from build123d import *

# Parameters (mm, degrees)
SKETCH1_W           = 50
SKETCH1_H           = 51
BOSS_EXTRUDE1_DEPTH = 3
SKETCH2_W           = 50
SKETCH2_H           = 3
BOSS_EXTRUDE2_DEPTH = 50
FILLET1_R           = 2
CHAMFER1_SIZE       = 5
CUT_EXTRUDE1_DEPTH  = 50
SKETCH4_R           = 12.55
SKETCH4_R_2         = 2.1
CUT_EXTRUDE2_DEPTH  = 50
BOSS_EXTRUDE3_DEPTH = 3


with BuildPart() as part:
    # Sketch1 → Boss-Extrude1 (new body)
    with BuildSketch(Plane.XY):
        Rectangle(SKETCH1_W, SKETCH1_H)
    extrude(amount=BOSS_EXTRUDE1_DEPTH)

    # Sketch2 → Boss-Extrude2 (add)
    with BuildSketch(Plane.XY.offset(3)):
        with Locations((0, -24)):
            Rectangle(SKETCH2_W, SKETCH2_H)
    extrude(amount=BOSS_EXTRUDE2_DEPTH)

    # Fillet1
    fillet1_edges = [part.edges().sort_by_distance(p)[0] for p in [
        (0, -22.5, 3),
        (0, -25.5, 0),
    ]]
    fillet(fillet1_edges, radius=FILLET1_R)

    # Chamfer1
    chamfer1_edges = [part.edges().sort_by_distance(p)[0] for p in [
        (-25, -24, 53),
        (25, -24, 53),
        (-25, 25.5, 1.5),
        (25, 25.5, 1.5),
    ]]
    chamfer(chamfer1_edges, length=CHAMFER1_SIZE)

    # Sketch3 → Cut-Extrude1 (cut)
    with BuildSketch(Plane(origin=(0, -22.5, 0), x_dir=(1, 0, 0), z_dir=(0, 1, 0))):
        with BuildLine():
            Line((-17.1, -42), (-17.1, -12))
            ThreePointArc((-17.1, -12), (-15, -9.9), (-12.9, -12))
            Line((-12.9, -12), (-12.9, -42))
            ThreePointArc((-12.9, -42), (-15, -44.1), (-17.1, -42))
        make_face()
        with BuildLine():
            Line((12.9, -42), (12.9, -12))
            ThreePointArc((12.9, -12), (15, -9.9), (17.1, -12))
            Line((17.1, -12), (17.1, -42))
            ThreePointArc((17.1, -42), (15, -44.1), (12.9, -42))
        make_face()
    extrude(amount=-CUT_EXTRUDE1_DEPTH, mode=Mode.SUBTRACT)

    # Sketch4 → Cut-Extrude2 (cut)
    with BuildSketch(Plane.XY.offset(3)):
        with Locations((0, 4.5)):
            Circle(SKETCH4_R)
        with Locations((0, 22)):
            Circle(SKETCH4_R_2)
        with Locations((0, -13)):
            Circle(SKETCH4_R_2)
        with Locations((17.5, 4.5)):
            Circle(SKETCH4_R_2)
        with Locations((-17.5, 4.5)):
            Circle(SKETCH4_R_2)
    extrude(amount=-CUT_EXTRUDE2_DEPTH, mode=Mode.SUBTRACT)

    # Sketch5 → Boss-Extrude3 (add)
    with BuildSketch(Plane.ZY.offset(25)):
        with BuildLine():
            Line((3, -2.5), (16, -22.5))
            Line((16, -22.5), (5, -22.5))
            ThreePointArc((5, -22.5), (3.585786438, -21.914213562), (3, -20.5))
            Line((3, -20.5), (3, -2.5))
        make_face()
    boss_extrude3 = extrude(amount=-BOSS_EXTRUDE3_DEPTH)

    # Mirror1: Boss-Extrude3 across plane
    add(boss_extrude3.mirror(Plane(origin=(0, 0, 0), x_dir=(0, 0, 1), z_dir=(1, 0, 0))))


solid = part.part
Geometry: final body of the model. Coordinates: model frame, mm. A direction names the side the tool comes from. Give positions to 0.01 mm unless a question says otherwise; leave off trailing zeros. Write each loop counter-clockwise with the first axis right and the second up, starting at its lowest first coordinate (ties: lowest second). Pieces come first, ordered by that corner, then holes. Notation, with made-up numbers: M 67.5,29.25 L 77.5,29.25 A25 cw 77.5,53.25 Z; hole C 60,-1.75 d1. An arc over 180 degrees is marked long. Answer in a Markdown table with one row per item. Add a question column.
(1) First-contact query: pin 1 (10.5 mm diameter, centred on y = -9, z = 11.5, fed in from +X); pin 2 (5 mm diameter, centred on x = -9, z = 45, fed in from +Y); pin 3 (6.5 mm diameter, centred on x = 17.5, y = 4.5, fed in from +Z); pin 4 (3.5 mm diameter, centred on x = 0, y = -13, fed in from -Z). Flat tips, straight axial feed; report the tip coordinate or a pass-through.
(2) Ray query, line 1 (Y direction, x = 0, z = 2); line 2 (Y direction, x = 5.5, z = 26); line 3 (Z direction, x = 0.5, y = 19.5). Return the intervals inside material, ascending.
(3) Reachability of faces 1 (the cylindrical face through (0.31, -21.9, 3.57)), 2 (the flat face through (-22, -24, 51)), 3 (the flat face through (17.1, -24, 27)) from +Z, -Z, +X, -X, +Y, -Y: full face, straight path, thin tool, end or side. Return the list, or none.
(4) Section D-D on y = 4.5. Return loops of the section in (x, z).
(5) Mould query, pull axis X, two halves, no side actions, for faces 4 (the cylindrical face through (-0.273, -10.918, 1.521)), 5 (the flat face through (-22.5, 23, 1.5)), 6 (the flat face through (23, -24, 50)), 7 (the flat face through (22, -17, 7)). Classes: +X half, -X half, draft (parallel to the pull), parting line (faces both ways), or undercut.
(6) Section B-B on y = 22. Return loops of the section in (x, z), and give its area (3 significant figures).
(7) Section A-A on z = 35. Return loops of the section in (x, y), and give its area (3 significant figures).
(8) Section C-C on x = 10. Return loops of the section in (y, z).
Result set:
| question | item | result |
|---|---|---|
| 1 | pin 1 | stops at x = 25 |
| 1 | pin 2 | stops at y = -22.5 |
| 1 | pin 3 | stops at z = 3 |
| 1 | pin 4 | passes through |
| 2 | line 1 | y = -25.5 to -15.1, -10.9 to -8.05, 17.05 to 19.9, 24.1 to 25.5 |
| 2 | line 2 | y = -25.5 to -22.5 |
| 2 | line 3 | z = 0 to 3 |
| 3 | face 1 | +Z, +Y |
| 3 | face 2 | +Z, -X, +Y, -Y |
| 3 | face 3 | +Y, -Y |
| 4 | outline | M -25,0 L -19.6,0 L -19.6,3 L -25,3 Z; M -15.4,0 L -12.55,0 L -12.55,3 L -15.4,3 Z; M 12.55,0 L 15.4,0 L 15.4,3 L 12.55,3 Z; M 19.6,0 L 25,0 L 25,3 L 19.6,3 Z |
| 5 | face 4 | undercut |
| 5 | face 5 | -X half |
| 5 | face 6 | +X half |
| 5 | face 7 | undercut |
| 6 | outline | M -23.5,0 L -2.1,0 L -2.1,3 L -23.5,3 Z; M 2.1,0 L 23.5,0 L 23.5,3 L 2.1,3 Z |
| 6 | area | 128 mm^2 |
| 7 | outline | M -25,-25.5 L -17.1,-25.5 L -17.1,-22.5 L -25,-22.5 Z; M -12.9,-25.5 L 12.9,-25.5 L 12.9,-22.5 L -12.9,-22.5 Z; M 17.1,-25.5 L 25,-25.5 L 25,-22.5 L 17.1,-22.5 Z |
| 7 | area | 125 mm^2 |
| 8 | outline | M -25.5,2 A2 ccw -23.5,0 L -3.08,0 L -3.08,3 L -20.5,3 A2 cw -22.5,5 L -22.5,53 L -25.5,53 Z; M 12.08,0 L 25.5,0 L 25.5,3 L 12.08,3 Z |
